```python
from build123d import *

# Parameters (mm, degrees)
F0_R     = 7.5
F1_DEPTH = 16
F3_W     = 12
F3_H     = 39.696938
F3_H_2   = 10.303062
F4_DEPTH = 40.001
F5_R     = 4


with BuildPart() as f1:
    # F0 (on Front) → F1 (new body, symmetric)
    with BuildSketch(Plane.XZ):
        with BuildLine():
            Line((15, -86), (15, 0))
            ThreePointArc((15, 0), (-11.61895, 9.486833), (3, -14.696938))
            Line((3, -14.696938), (3, -86))
            Line((3, -86), (15, -86))
        make_face()
        Circle(F0_R, mode=Mode.SUBTRACT)
    extrude(amount=F1_DEPTH, both=True)

    # F3 (on offset) → F4 (cut, through all)
    with BuildSketch(Plane.YZ.offset(-25)):
        with Locations((0, 5.151531)):
            Rectangle(F3_W, F3_H)
        with Locations((0, -19.848469)):
            Rectangle(F3_W, F3_H_2)
        with BuildLine():
            ThreePointArc((0, -86), (-11.313709, -81.313708), (-16, -70))
            Line((-16, -70), (-16, -86))
            Line((-16, -86), (0, -86))
        make_face()
        with BuildLine():
            Line((16, -86), (16, -70))
            ThreePointArc((16, -70), (11.313708, -81.313709), (0, -86))
            Line((0, -86), (16, -86))
        make_face()
        with BuildLine():
            Line((6, -70), (6, -45))
            ThreePointArc((6, -45), (0, -39), (-6, -45))
            Line((-6, -45), (-6, -70))
            ThreePointArc((-6, -70), (0, -76), (6, -70))
        make_face()
    extrude(amount=F4_DEPTH, mode=Mode.SUBTRACT)

    # F5
    f5_edges = [f1.edges().sort_by_distance(p)[0] for p in [
        (3, 11, -14.696938),
        (3, -11, -14.696938),
    ]]
    fillet(f5_edges, radius=F5_R)


solid = f1.part
```
Read the model definition and answer for the solid it produces. Units are mm, in the model's axes. A direction names the side the tool comes from. Coordinates: 2 decimals unless noted, no trailing zeros. Loops run counter-clockwise (first coordinate to the right, second up) from the corner with the lowest first, then second, coordinate; pieces in that order, holes last. Notation, with made-up numbers: (68, 32.25) -> (89, 32.25) arc R21 ccw to (89, 37.25) -> close; hole circle Ø1 at (16.25, 86). An arc over 180 degrees is marked (long way). Return JSON: item names as keys, results as strings.
Item 1: Find section D-D (y = -8). Determine the outline of the cut face in (x, z).
Answers:
{"outline": "(-0.79, -14.98) arc R4 cw to (3, -18.97) -> (3, -83.86) -> (15, -83.86) -> (15, 0) arc R15 ccw (long way) to start; hole circle Ø15 at (0, 0)"}
Item 2: Flat-ended cylindrical pins translate along their axes: P1, Ø12, axis at x = 6.5, y = 5.5, coming from the -Z side; P2, Ø6, axis at x = 7.5, y = -1.5, coming from the +Z side; P3, Ø9.5, axis at y = 4.5, z = -66.5, coming from the -X side; P4, Ø8, axis at x = 2, y = 10, coming from the -Z side. Find the tip coordinate at first contact, or state that the pin passes through.
Answers:
{"P1": "stops at z = -86", "P2": "stops at z = -25", "P3": "stops at x = 3", "P4": "stops at z = -84.78"}
Item 3: Find the intervals of material crossed by probe 1 along X at (y, z) = (12, 0); probe 2 along Y at (x, z) = (3, -14); probe 3 along X at (y, z) = (14.5, -54.5), in increasing order.
Answers:
{"probe 1": "x = -15 to -7.5, 7.5 to 15", "probe 2": "y = -16 to -6, 6 to 16", "probe 3": "x = 3 to 15"}
Item 4: For a pull along Z with two mould halves and no side action, classify faces 1 (the cylindrical face through (9, 0, -76)), 2 (the cylindrical face through (1.87, -11.07, -16.19)), 3 (the flat face through (6, -6, -5)), 4 (the cylindrical face through (-7.493, -10.93, 0.33)) as +Z half, -Z half, draft (parallel to the pull), parting line (faces both ways), or undercut.
Answers:
{"face 1": "undercut", "face 2": "-Z half", "face 3": "draft", "face 4": "undercut"}
Item 5: Find section A-A (x = 4.75). Determine the outline of the cut face in (y, z).
Answers:
{"outline": "(-16, -70) arc R16 ccw to (16, -70) -> (16, -5.8) -> (6, -5.8) -> (6, -25) -> (-6, -25) -> (-6, -5.8) -> (-16, -5.8) -> close; (-16, 5.8) -> (-6, 5.8) -> (-6, 14.23) -> (-16, 14.23) -> close; (6, 5.8) -> (16, 5.8) -> (16, 14.23) -> (6, 14.23) -> close; hole (-6, -70) arc R6 ccw to (6, -70) -> (6, -45) arc R6 ccw to (-6, -45) -> close"}
Item 6: For faces 5 (the flat face through (6, 6, -5)), 6 (the flat face through (3, 7, -52)), 7 (the flat face through (9, -6, -57)), 8 (the cylindrical face through (-7.493, 11.07, 0.33)), 9 (the flat face through (6, 16, -27)), determine the directions among +Z, -Z, +X, -X, +Y, -Y from which every point of the face is accessible in a straight line to the end or side of a thin tool.
Answers:
{"face 5": "+Z, +X, -X", "face 6": "-Z, -X, +Y, -Y", "face 7": "+X, -X", "face 8": "+Y, -Y", "face 9": "+Z, -Z, +X, -X, +Y"}
Item 7: Find section B-B (z = -23.5). Determine the outline of the cut face in (x, y).
Answers:
{"outline": "(3, -16) -> (15, -16) -> (15, -6) -> (3, -6) -> close; (3, 6) -> (15, 6) -> (15, 16) -> (3, 16) -> close"}
Item 8: Find section C-C (x = -10.25). Determine the outline of the cut face in (y, z).
Answers:
{"outline": "(-16, -10.95) -> (-6, -10.95) -> (-6, 10.95) -> (-16, 10.95) -> close; (6, -10.95) -> (16, -10.95) -> (16, 10.95) -> (6, 10.95) -> close"}
